```python
from build123d import *

# Parameters (mm, degrees)
F1_DEPTH    = 63.5
F2_DEPTH    = 25.4
F3_DEPTH    = 7.9375
F5_T1_DEPTH = 7.9375
F5_T3_DEPTH = 7.9375
F5_T8_DEPTH = 8.0594365629


# Not quite as in the source:
# - a fillet or chamfer that OpenCascade refuses, or shapes differently, is made with other operations: its cross-section is extruded or revolved along the edge and cut away or added


with BuildPart() as f1:
    # F0 (on Front) → F1 (new body, symmetric)
    with BuildSketch(Plane.XZ):
        Polygon((-41.275, 9.525), (-41.275, -9.525), (41.275, -9.525), (41.275, 9.525), (22.2249999642, 9.525), align=None)
    extrude(amount=F1_DEPTH, both=True)

    # F0 (on Front) → F2 (join, symmetric)
    with BuildSketch(Plane.XZ):
        with BuildLine():
            Line((22.2249999642, 9.525), (41.275, 9.525))
            Line((41.275, 9.525), (41.275, 27.0002))
            ThreePointArc((41.275, 27.0002), (45.9246798487, 38.2255201513), (57.15, 42.8752))
            Line((57.15, 42.8752), (60.325, 42.8752))
            Line((60.325, 42.8752), (60.325, 61.9252000358))
            Line((60.325, 61.9252000358), (57.15, 61.9252000358))
            ThreePointArc((57.15, 61.9252000358), (32.4542956418, 51.6959043582), (22.2249999642, 27.0002))
            Line((22.2249999642, 27.0002), (22.2249999642, 9.525))
        make_face()
        Polygon((85.8965185289, 61.9252000358), (60.325, 61.9252000358), (60.325, 42.8752), (85.759376848, 42.8752), align=None)
    extrude(amount=F2_DEPTH, both=True)

    # F0 (on Front) → F3 (join, symmetric)
    with BuildSketch(Plane.XZ):
        with BuildLine():
            add(Edge.make_bspline(
                [(-41.275, 9.525), (-42.0210659504, 47.4507585168), (0, 63.975892961), (57.15, 61.9252000358)],
                knots=[0, 0, 0, 0, 111.5045361803, 111.5045361803, 111.5045361803, 111.5045361803], degree=3))
            Line((-41.275, 9.525), (22.2249999642, 9.525))
            Line((22.2249999642, 9.525), (22.2249999642, 27.0002))
            ThreePointArc((22.2249999642, 27.0002), (32.4542956418, 51.6959043582), (57.15, 61.9252000358))
        make_face()
    extrude(amount=F3_DEPTH, both=True)

    # F0 (on Front) → F4 (revolve)
    with BuildSketch(Plane.XZ):
        Polygon((85.9307125211, 66.675), (85.8965185289, 61.9252000358), (85.759376848, 42.8752), (85.725, 38.1), (111.125, 38.1), (111.125, 66.675), align=None)
    revolve(axis=Axis((85.8278562605, 0, 52.3875), (0.0071988518, 0, 0.9999740879)))

    # F5: fillet of radius 5.08 on 6 edges, made by hand

    # F5_s2 → F5_t1 (join)
    with BuildSketch(Plane.XZ):
        with BuildLine():
            ThreePointArc((57.0602012116, 61.9284074084), (57.1504319335, 61.9260019422), (57.2406911513, 61.9252000358))
            Line((57.2406911513, 61.9252000358), (57.2406911513, 61.8236000358))
            Line((57.2406911513, 61.8236000358), (57.15, 61.8236000358))
            Line((57.15, 61.8236000358), (57.1463566684, 61.8236653809))
            ThreePointArc((57.1463566684, 61.8236653809), (57.1014741691, 61.8252721742), (57.0565914128, 61.8268715558))
            Line((57.0565914128, 61.8268715558), (57.0602012116, 61.9284074084))
        make_face()
    extrude(amount=F5_T1_DEPTH)

    # F5_s4 → F5_t3 (join)
    with BuildSketch(Plane.XZ.offset(-7.9375)):
        with BuildLine():
            ThreePointArc((57.0602012116, 61.9284074084), (57.1504319335, 61.9260019422), (57.2406911513, 61.9252000358))
            Line((57.2406911513, 61.9252000358), (57.2406911513, 61.8236000358))
            Line((57.2406911513, 61.8236000358), (57.15, 61.8236000358))
            Line((57.15, 61.8236000358), (57.1463566684, 61.8236653809))
            ThreePointArc((57.1463566684, 61.8236653809), (57.1014741691, 61.8252721742), (57.0565914128, 61.8268715558))
            Line((57.0565914128, 61.8268715558), (57.0602012116, 61.9284074084))
        make_face()
    extrude(amount=F5_T3_DEPTH)


with BuildPart() as f5_tool6:
    # F5_s7 → F5_t8 (new body)
    with BuildSketch(Plane.XZ.offset(0.1219365629)):
        with BuildLine():
            ThreePointArc((-41.275, 9.4762253748), (-41.2752233916, 9.5238657859), (-41.2758935468, 9.5715020071))
            Line((-41.2758935468, 9.5715020071), (-41.1743114177, 9.5734075397))
            ThreePointArc((-41.1743114177, 9.5734075397), (-41.1738708312, 9.5502028132), (-41.1734196528, 9.526998263))
            Line((-41.1734196528, 9.526998263), (-41.1734, 9.525))
            Line((-41.1734, 9.525), (-41.1734, 9.4762253748))
            Line((-41.1734, 9.4762253748), (-41.275, 9.4762253748))
        make_face()
    extrude(amount=-F5_T8_DEPTH)

    split(bisect_by=Plane.XY.offset(9.525), keep=Keep.BOTTOM)


with BuildPart() as f1_1:
    add(f1.part)

    # F5_t5: union F5_tool6
    add(f5_tool6.part)


solid = f1_1.part
```
Verification items for the finished model (mm, model axes). A direction names the side the tool comes from. Coordinates: 2 decimals unless noted, no trailing zeros. Loops run counter-clockwise (first coordinate to the right, second up) from the corner with the lowest first, then second, coordinate; pieces in that order, holes last. Notation, with made-up numbers: (79.25, -14.5) -> (127.25, -14.5) arc R13 ccw to (127.25, 4.5) -> close; hole circle Ø10 at (37, 30). An arc over 180 degrees is marked (long way). Put each result on its own line as item: value.
1. Thickness scan on line 1 (Z direction, x = 40, y = -58) (3 decimals); line 2 (X direction, y = -28.5, z = -5.5) (3 decimals); line 3 (Z direction, x = 88, y = 3). Record the ranges inside material, lowest first.
Result set:
line 1: z = -9.525 to 9.525
line 2: x = -41.275 to 41.275
line 3: z = 38.11 to 66.69
2. Section check B-B, the plane z = -3.5. Record the boundary of the cut face in (x, y) (3 decimals).
Result set:
outline: (-41.275, -63.5) -> (41.275, -63.5) -> (41.275, 63.5) -> (-41.275, 63.5) -> close
3. Gauge pin test, flat ends, axial feed: P1, Ø12, axis at x = -21.5, y = -25.5, coming from the +Z side (3 decimals); P2, Ø9.5, axis at y = -20, z = -2.5, coming from the -X side (3 decimals); P3, Ø4, axis at x = 94.5, z = 44.5, coming from the -Y side. Record the tip position at first contact, or that the pin passes through.
Result set:
P1: stops at z = 9.525
P2: stops at x = -41.275
P3: stops at y = -24.45
4. Mould release check, pull along X, two halves, no side actions. Record for faces 6 (the face through (22.225, 17, 18)), 7 (the face through (87.2, -0.6, 38.1)), 8 (the face through (1, -36, 9.525)), 9 (the face through (60, 0, 61.925)): pulls with the +X half, pulls with the -X half, needs draft (parallel to the pull), parting line crosses it, or undercut.
Result set:
face 6: pulls with the -X half
face 7: undercut
face 8: needs draft
face 9: undercut
5. Section check A-A, the plane y = -55. Record the boundary of the cut face in (x, z) (3 decimals), then the cut area to 3 significant figures.
Result set:
outline: (-41.275, -9.525) -> (41.275, -9.525) -> (41.275, 9.525) -> (-41.275, 9.525) -> close
area: 1,570 mm^2
6. Tool access check on faces 1 (the face through (47, 25.4, 42)), 2 (the face through (47, -25.4, 42)), 3 (the face through (1, 35, 9.525)), 4 (the face through (41.275, -1, 4)), 5 (the face through (45.8, -0.4, 38.1)). Record the directions out of +Z, -Z, +X, -X, +Y, -Y that give a thin tool (end or side, any length) a straight path to the whole face; none if there is none.
Result set:
face 1: +Z, +X, -X, +Y
face 2: +Z, +X, -X, -Y
face 3: +Z, -X, +Y
face 4: -Z, +X, +Y, -Y
face 5: -Z, +Y, -Y
